The figure shows three views and two pictorial views of one solid part (mm, origin at its lowest corner). Answer the questions. Round coordinates to 2 decimals unless told otherwise and drop trailing zeros. Order: outer loops, then holes, each group sorted by start corner. A loop starts at its lowest first (then second) coordinate and runs counter-clockwise, first axis right, second up. Notation, with made-up numbers: (16.5, -9.5) - (41.5, -9.5) arc R15 ccw to (41.5, 9.5) - close; hole circle Ø7 at (27.5, 33). An arc over 180 degrees is marked (long way). One line per item, written item: value. Start each with the question number.
1. Section A-A, the plane x = 20.5 is taken. Give the vertices of the cut face in (y, z), then the cut area to 3 significant figures.
2. Section B-B, the plane y = 1.3 is taken. Give the vertices of the cut face in (x, z), then the cut area to 3 significant figures.
3. Straight lines are drawn through the part: line 1 (Z direction, x = 17, y = 4.25); line 2 (X direction, y = 1.55, z = 36.5); line 3 (Z direction, x = 11, y = 4.35). For each, find the intervals that lie inside material, in ascending order.
4. Section C-C, the plane z = 21 is taken. Give the vertices of the cut face in (x, y), then the cut area to 3 significant figures.
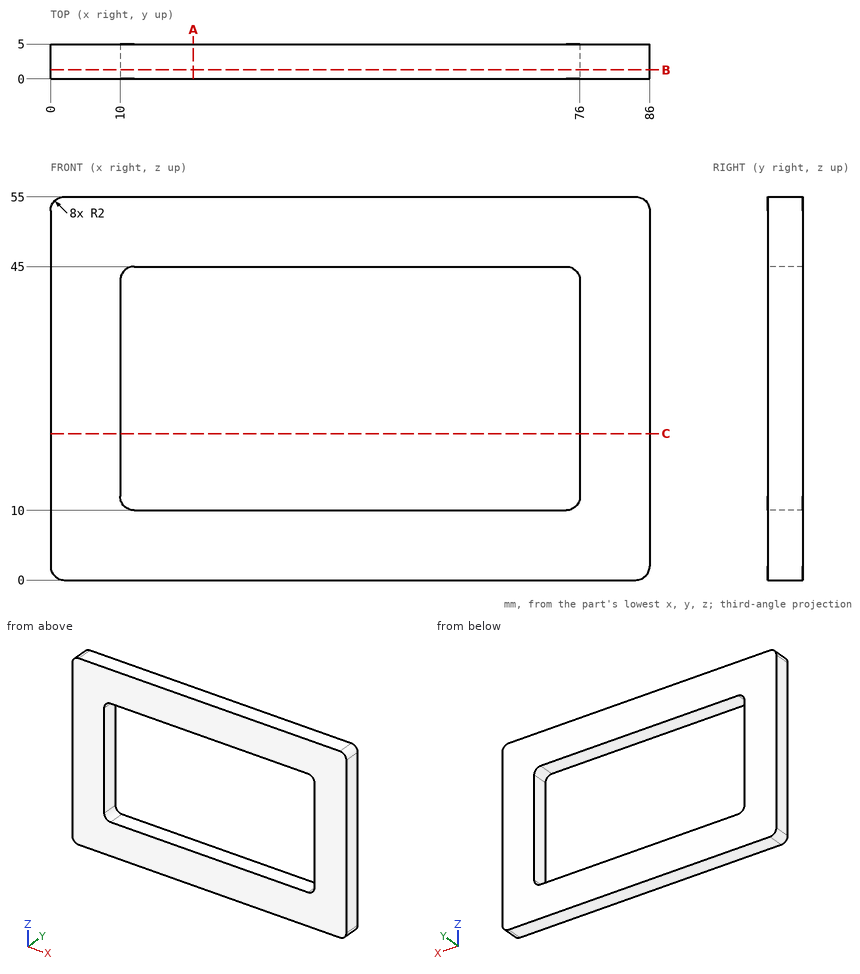
Answer list:
1. outline: (0, 0) - (5, 0) - (5, 10) - (0, 10) - close; (0, 45) - (5, 45) - (5, 55) - (0, 55) - close
1. area: 100 mm²
2. outline: (0, 2) arc R2 ccw to (2, 0) - (84, 0) arc R2 ccw to (86, 2) - (86, 53) arc R2 ccw to (84, 55) - (2, 55) arc R2 ccw to (0, 53) - close; hole (10, 12) arc R2 ccw to (12, 10) - (74, 10) arc R2 ccw to (76, 12) - (76, 43) arc R2 ccw to (74, 45) - (12, 45) arc R2 ccw to (10, 43) - close
2. area: 2,420 mm²
3. line 1: z = 0 to 10, 45 to 55
3. line 2: x = 0 to 10, 76 to 86
3. line 3: z = 0 to 10.27, 44.73 to 55
4. outline: (0, 0) - (10, 0) - (10, 5) - (0, 5) - close; (76, 0) - (86, 0) - (86, 5) - (76, 5) - close
4. area: 100 mm²
